For this review, take the finished solid that the model builds, in its own axes (mm). Face numbers are marked on the shaded views. A direction names the side the tool comes from. Coordinates: 2 decimals unless noted, no trailing zeros. Loops run counter-clockwise (first coordinate to the right, second up) from the corner with the lowest first, then second, coordinate; pieces in that order, holes last. Notation, with made-up numbers: M -37.75,-20.5 L -26.75,-20.5 A31 cw -26.75,8.5 Z; hole C 41,-11 d9. An arc over 180 degrees is marked long. Answer as a JSON object with one key per item and string values. Group by question number.
Item 1: Add section A-A (x = -7.3). State the section outline as (y, z) points (3 decimals).
Item 2: Insertion check: pin 1 (4 mm diameter, centred on x = -20, z = 27, fed in from +Y); pin 2 (10 mm diameter, centred on x = -13, y = -26, fed in from +Z); pin 3 (3 mm diameter, centred on y = -5, z = 7.5, fed in from +X). Each pin has a flat end and moves straight along its axis. Give the tip position at first contact, or say it passes through.
Item 3: Wall thickness on L1, parallel to X at y = -53.5, z = 29.94 (3 decimals); L2, parallel to Z at x = -32.73, y = -53.5 (3 decimals); L3, parallel to X at y = -17.5, z = 2: over which ranges is each line inside the solid? List them lowest first. Write a range as from..to.
Item 4: Add section D-D (x = -32.73). State the section outline as (y, z) points (3 decimals).
Item 5: Add section C-C (z = 12). State the section outline as (x, y) points, then the cut area to 3 significant figures.
Item 6: Tool access review of the marked faces 4, 5, 6, 7 and 8: name each direction out of +Z, -Z, +X, -X, +Y, -Y from which nothing blocks a thin tool from reaching the whole face with its end or side.
Item 7: Mouldability with a two-part tool opening along Z and no side actions: class the marked faces 1, 2 and 3 as +Z half, -Z half, draft (parallel to the pull), parting line (faces both ways), or undercut.
Item 8: Add section B-B (y = -27). State the section outline as (x, z) points.
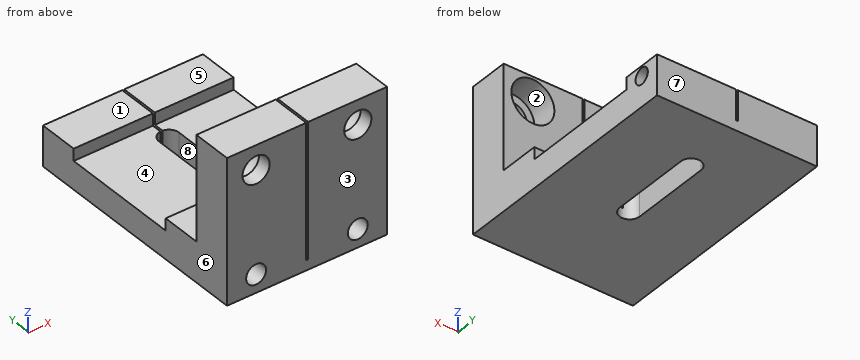
from build123d import *

# Parameters (mm, degrees)
SKETCH1_W           = 40
SKETCH1_H           = 60
BOSS_EXTRUDE1_DEPTH = 10
CUT_EXTRUDE1_DEPTH  = 11
SKETCH5_W           = 3
SKETCH5_H           = 30
CUT_EXTRUDE4_DEPTH  = 41
SKETCH6_W           = 40
SKETCH6_H           = 10
BOSS_EXTRUDE2_DEPTH = 26
SKETCH8_W           = 0.5
SKETCH8_H           = 33.5
CUT_EXTRUDE7_DEPTH  = 60
SKETCH10_R          = 2
CUT_EXTRUDE10_DEPTH = 30
SKETCH12_R          = 3.4
SKETCH12_R_2        = 2.49
CUT_EXTRUDE13_DEPTH = 10
SKETCH14_R          = 5.375
CUT_EXTRUDE14_DEPTH = 6.5


with BuildPart() as part:
    # Sketch1 → Boss-Extrude1 (new body)
    with BuildSketch(Plane.XY):
        with Locations((-20, -30)):
            Rectangle(SKETCH1_W, SKETCH1_H)
    extrude(amount=BOSS_EXTRUDE1_DEPTH)

    # Sketch2 → Cut-Extrude1 (cut, through all)
    with BuildSketch(Plane.XY.offset(10)):
        with BuildLine():
            Line((-17.5, -15), (-17.5, -35))
            ThreePointArc((-17.5, -35), (-20, -37.5), (-22.5, -35))
            Line((-22.5, -35), (-22.5, -15))
            ThreePointArc((-22.5, -15), (-20, -12.5), (-17.5, -15))
        make_face()
    extrude(amount=-CUT_EXTRUDE1_DEPTH, mode=Mode.SUBTRACT)

    # Sketch5 → Cut-Extrude4 (cut, through all)
    with BuildSketch(Plane(origin=(0, 0, 0), x_dir=(0, 0, -1), z_dir=(1, 0, 0))):
        with Locations((-8.5, -25)):
            Rectangle(SKETCH5_W, SKETCH5_H)
    extrude(amount=-CUT_EXTRUDE4_DEPTH, mode=Mode.SUBTRACT)

    # Sketch6 → Boss-Extrude2 (add)
    with BuildSketch(Plane.XY.offset(10)):
        with Locations((-20, -55)):
            Rectangle(SKETCH6_W, SKETCH6_H)
    extrude(amount=BOSS_EXTRUDE2_DEPTH)

    # Sketch8 → Cut-Extrude7 (cut)
    with BuildSketch(Plane(origin=(0, 0, 0), x_dir=(1, 0, 0), z_dir=(0, 1, 0))):
        with Locations((-19.95, -19.25)):
            Rectangle(SKETCH8_W, SKETCH8_H)
    extrude(amount=-CUT_EXTRUDE7_DEPTH, mode=Mode.SUBTRACT)

    # Sketch10 → Cut-Extrude10 (cut)
    with BuildSketch(Plane(origin=(0, 0, 0), x_dir=(0, 0, -1), z_dir=(1, 0, 0))):
        with Locations((-7.5, -5)):
            Circle(SKETCH10_R)
    extrude(amount=-CUT_EXTRUDE10_DEPTH, mode=Mode.SUBTRACT)

    # Sketch12 → Cut-Extrude13 (cut)
    with BuildSketch(Plane.XZ.offset(60)):
        with Locations((-7.3, 29.94)):
            Circle(SKETCH12_R)
        with Locations((-32.73, 29.94)):
            Circle(SKETCH12_R)
        with Locations((-32.73, 4.51)):
            Circle(SKETCH12_R_2)
        with Locations((-7.3, 4.51)):
            Circle(SKETCH12_R_2)
    extrude(amount=-CUT_EXTRUDE13_DEPTH, mode=Mode.SUBTRACT)

    # Sketch14 → Cut-Extrude14 (cut)
    with BuildSketch(Plane(origin=(0, -50, 0), x_dir=(1, 0, 0), z_dir=(0, 1, 0))):
        with Locations((-32.73, -29.94)):
            Circle(SKETCH14_R)
        with Locations((-7.3, -29.94)):
            Circle(SKETCH14_R)
    extrude(amount=-CUT_EXTRUDE14_DEPTH, mode=Mode.SUBTRACT)


solid = part.part
From the geometry:
{
 "1": {"outline": "M -60,0 L 0,0 L 0,10 L -10,10 L -10,7 L -40,7 L -40,10 L -50,10 L -50,24.565 L -56.5,24.565 L -56.5,26.54 L -60,26.54 L -60,7 L -50,7 L -50,2.02 L -60,2.02 Z; M -60,33.34 L -56.5,33.34 L -56.5,35.315 L -50,35.315 L -50,36 L -60,36 Z; hole C -5,7.5 d4"},
 "2": {"pin 1": "stops at y = -50", "pin 2": "stops at z = 7", "pin 3": "stops at x = -30"},
 "3": {"L1": "x = -40..-38.105, -27.355..-20.2, -19.7..-12.675, -1.925..0", "L2": "z = 0..2.02, 7..24.565, 35.315..36", "L3": "x = -40..-22.5, -17.5..0"},
 "4": {"outline": "M -60,0 L 0,0 L 0,10 L -10,10 L -10,7 L -40,7 L -40,10 L -50,10 L -50,24.565 L -56.5,24.565 L -56.5,26.54 L -60,26.54 L -60,7 L -50,7 L -50,2.02 L -60,2.02 Z; M -60,33.34 L -56.5,33.34 L -56.5,35.315 L -50,35.315 L -50,36 L -60,36 Z"},
 "5": {"outline": "M -40,-60 L -20.2,-60 L -20.2,-50 L -40,-50 Z; M -19.7,-60 L 0,-60 L 0,-50 L -19.7,-50 Z", "area": "395 mm²"},
 "6": {"face 4": "+Z, +X, -X", "face 5": "+Z, +X, -X, +Y", "face 6": "+Z, -Z, -X, +Y, -Y", "face 7": "+Z, -Z, +X, -X, +Y", "face 8": "+Z, -Z"},
 "7": {"face 1": "+Z half", "face 2": "undercut", "face 3": "draft"},
 "8": {"outline": "M -40,0 L -22.5,0 L -22.5,7 L -40,7 Z; M -17.5,0 L 0,0 L 0,7 L -17.5,7 Z"}
}
